Model file for the job. Use its own axes, mm. Face numbers are marked on the shaded views. A direction names the side the tool comes from. Give positions to 0.01 mm unless a question says otherwise; leave off trailing zeros. Loops run counter-clockwise (first coordinate to the right, second up) from the corner with the lowest first, then second, coordinate; pieces in that order, holes last. Notation, with made-up numbers: M -33.5,12.25 L -17.5,12.25 A20 ccw -17.5,33.25 Z; hole C -12,44.5 d10. An arc over 180 degrees is marked long. Answer in a Markdown table with one row per item.
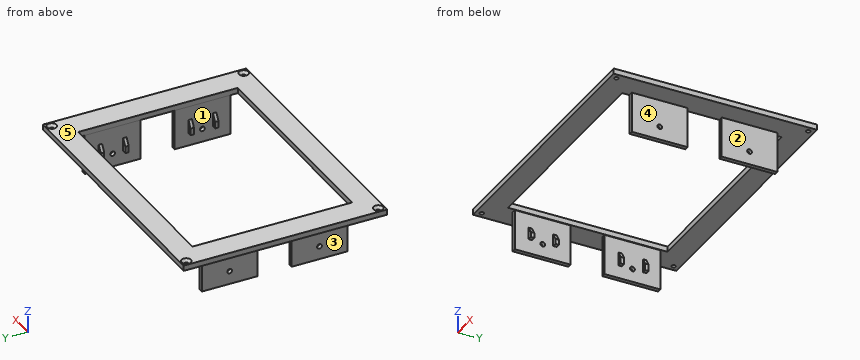
```python
from build123d import *
from OCP.BRepFilletAPI import BRepFilletAPI_MakeChamfer

# Parameters (mm, degrees)
ESQUISSE1_W             = 197
ESQUISSE1_H             = 149.5
BOSS_EXTRU_1_DEPTH      = 4
ESQUISSE3_R             = 1.5
ENL_V_MAT_EXTRU_2_DEPTH = 4
CHANFREIN1_SIZE         = 2
ESQUISSE4_W             = 160
ESQUISSE4_H             = 117.3
ENL_V_MAT_EXTRU_3_DEPTH = 10
ESQUISSE5_W             = 3
ESQUISSE5_H             = 41
BOSS_EXTRU_2_DEPTH      = 30
ESQUISSE6_W             = 10
ESQUISSE6_H             = 2.5
ESQUISSE6_W_2           = 8.882781921
BOSS_EXTRU_3_DEPTH      = 3
ESQUISSE7_W             = 10
ESQUISSE7_H             = 2.5
BOSS_EXTRU_4_DEPTH      = 3
CHANFREIN2_SIZE         = 3
CHANFREIN2_SIZE_2       = 5
ESQUISSE8_R             = 1.75
ENL_V_MAT_EXTRU_4_DEPTH = 210


with BuildPart() as part:
    # Esquisse1 → Boss.-Extru.1 (new body)
    with BuildSketch(Plane.XY):
        with Locations((98.5, 74.75)):
            Rectangle(ESQUISSE1_W, ESQUISSE1_H)
    extrude(amount=BOSS_EXTRU_1_DEPTH)

    # Esquisse3 → Enlèv. mat.-Extru.2 (cut)
    with BuildSketch(Plane.XY.offset(4)):
        with Locations((4.25, 145.25)):
            Circle(ESQUISSE3_R)
        with Locations((4.25, 4.25)):
            Circle(ESQUISSE3_R)
        with Locations((192.75, 4.25)):
            Circle(ESQUISSE3_R)
        with Locations((192.75, 145.25)):
            Circle(ESQUISSE3_R)
    extrude(amount=-ENL_V_MAT_EXTRU_2_DEPTH, mode=Mode.SUBTRACT)

    # Chanfrein1
    chanfrein1_edges = [part.edges().sort_by_distance(p)[0] for p in [
        (2.75, 145.25, 4),
        (2.75, 4.25, 4),
        (191.25, 4.25, 4),
        (191.25, 145.25, 4),
    ]]
    chamfer(chanfrein1_edges, length=CHANFREIN1_SIZE)

    # Esquisse4 → Enlèv. mat.-Extru.3 (cut)
    with BuildSketch(Plane.XY.offset(4)):
        with Locations((98.25, 74.75)):
            Rectangle(ESQUISSE4_W, ESQUISSE4_H)
    extrude(amount=-ENL_V_MAT_EXTRU_3_DEPTH, mode=Mode.SUBTRACT)

    # Esquisse5 → Boss.-Extru.2 (add)
    with BuildSketch(Plane(origin=(0, 0, 0), x_dir=(-1, 0, 0), z_dir=(0, 0, -1))):
        with Locations((-180.25, 107.9)):
            Rectangle(ESQUISSE5_W, ESQUISSE5_H)
        with Locations((-180.25, 41.9)):
            Rectangle(ESQUISSE5_W, ESQUISSE5_H)
        with Locations((-16.25, 107.9)):
            Rectangle(ESQUISSE5_W, ESQUISSE5_H)
        with Locations((-16.25, 41.9)):
            Rectangle(ESQUISSE5_W, ESQUISSE5_H)
    extrude(amount=BOSS_EXTRU_2_DEPTH)

    # Esquisse6 → Boss.-Extru.3 (add)
    with BuildSketch(Plane(origin=(17.75, 0, 0), x_dir=(0, 0, -1), z_dir=(1, 0, 0))):
        with Locations((15.5, 116.9)):
            Rectangle(ESQUISSE6_W, ESQUISSE6_H)
        with Locations((15.5, 98.9)):
            Rectangle(ESQUISSE6_W, ESQUISSE6_H)
        with Locations((14.941390961, 50.9)):
            Rectangle(ESQUISSE6_W_2, ESQUISSE6_H)
        with Locations((14.941390961, 32.9)):
            Rectangle(ESQUISSE6_W_2, ESQUISSE6_H)
    extrude(amount=BOSS_EXTRU_3_DEPTH)

    # Esquisse7 → Boss.-Extru.4 (add)
    with BuildSketch(Plane.ZY.offset(-178.75)):
        with Locations((-15.5, 32.9)):
            Rectangle(ESQUISSE7_W, ESQUISSE7_H)
        with Locations((-15.5, 50.9)):
            Rectangle(ESQUISSE7_W, ESQUISSE7_H)
        with Locations((-15.5, 98.9)):
            Rectangle(ESQUISSE7_W, ESQUISSE7_H)
        with Locations((-15.5, 116.9)):
            Rectangle(ESQUISSE7_W, ESQUISSE7_H)
    extrude(amount=BOSS_EXTRU_4_DEPTH)

    # Chanfrein2
    chanfrein2_edges_1 = [part.edges().sort_by_distance(p)[0] for p in [
        (20.75, 98.9, -10.5),
    ]]
    chanfrein2_side_1 = [part.faces().sort_by_distance(p)[0] for p in [
        (20.69, 98.9, -10.5),
    ]]
    chanfrein2_edges_2 = [part.edges().sort_by_distance(p)[0] for p in [
        (20.75, 116.9, -10.5),
    ]]
    chanfrein2_side_2 = [part.faces().sort_by_distance(p)[0] for p in [
        (20.69, 116.9, -10.5),
    ]]
    chanfrein2_edges_3 = [part.edges().sort_by_distance(p)[0] for p in [
        (20.75, 32.9, -10.5),
    ]]
    chanfrein2_side_3 = [part.faces().sort_by_distance(p)[0] for p in [
        (20.69, 32.9, -10.5),
    ]]
    chanfrein2_edges_4 = [part.edges().sort_by_distance(p)[0] for p in [
        (20.75, 50.9, -10.5),
    ]]
    chanfrein2_side_4 = [part.faces().sort_by_distance(p)[0] for p in [
        (20.69, 50.9, -10.5),
    ]]
    chanfrein2_edges_5 = [part.edges().sort_by_distance(p)[0] for p in [
        (175.75, 116.9, -10.5),
    ]]
    chanfrein2_side_5 = [part.faces().sort_by_distance(p)[0] for p in [
        (175.81, 116.9, -10.5),
    ]]
    chanfrein2_edges_6 = [part.edges().sort_by_distance(p)[0] for p in [
        (175.75, 98.9, -10.5),
    ]]
    chanfrein2_side_6 = [part.faces().sort_by_distance(p)[0] for p in [
        (175.81, 98.9, -10.5),
    ]]
    chanfrein2_edges_7 = [part.edges().sort_by_distance(p)[0] for p in [
        (175.75, 50.9, -10.5),
    ]]
    chanfrein2_side_7 = [part.faces().sort_by_distance(p)[0] for p in [
        (175.81, 50.9, -10.5),
    ]]
    chanfrein2_edges_8 = [part.edges().sort_by_distance(p)[0] for p in [
        (175.75, 32.9, -10.5),
    ]]
    chanfrein2_side_8 = [part.faces().sort_by_distance(p)[0] for p in [
        (175.81, 32.9, -10.5),
    ]]
    chanfrein2 = BRepFilletAPI_MakeChamfer(part.part.solid().wrapped)
    for e in chanfrein2_edges_1:
        chanfrein2.Add(CHANFREIN2_SIZE - 0.0001, CHANFREIN2_SIZE_2 - 0.0001, e.wrapped, chanfrein2_side_1[0].wrapped)
    for e in chanfrein2_edges_2:
        chanfrein2.Add(CHANFREIN2_SIZE - 0.0001, CHANFREIN2_SIZE_2 - 0.0001, e.wrapped, chanfrein2_side_2[0].wrapped)
    for e in chanfrein2_edges_3:
        chanfrein2.Add(CHANFREIN2_SIZE - 0.0001, CHANFREIN2_SIZE_2 - 0.0001, e.wrapped, chanfrein2_side_3[0].wrapped)
    for e in chanfrein2_edges_4:
        chanfrein2.Add(CHANFREIN2_SIZE - 0.0001, CHANFREIN2_SIZE_2 - 0.0001, e.wrapped, chanfrein2_side_4[0].wrapped)
    for e in chanfrein2_edges_5:
        chanfrein2.Add(CHANFREIN2_SIZE - 0.0001, CHANFREIN2_SIZE_2 - 0.0001, e.wrapped, chanfrein2_side_5[0].wrapped)
    for e in chanfrein2_edges_6:
        chanfrein2.Add(CHANFREIN2_SIZE - 0.0001, CHANFREIN2_SIZE_2 - 0.0001, e.wrapped, chanfrein2_side_6[0].wrapped)
    for e in chanfrein2_edges_7:
        chanfrein2.Add(CHANFREIN2_SIZE - 0.0001, CHANFREIN2_SIZE_2 - 0.0001, e.wrapped, chanfrein2_side_7[0].wrapped)
    for e in chanfrein2_edges_8:
        chanfrein2.Add(CHANFREIN2_SIZE - 0.0001, CHANFREIN2_SIZE_2 - 0.0001, e.wrapped, chanfrein2_side_8[0].wrapped)
    add(Compound.cast(chanfrein2.Shape()), mode=Mode.REPLACE)  # a hair under: the kernel refuses the full size

    # Esquisse8 → Enlèv. mat.-Extru.4 (cut)
    with BuildSketch(Plane.ZY.offset(-14.75)):
        with Locations(Location((-20.25, 107.9, 0), (0, 0, 270))):
            Circle(ESQUISSE8_R)
        with Locations(Location((-20.25, 41.9, 0), (0, 0, 270))):
            Circle(ESQUISSE8_R)
    extrude(amount=-ENL_V_MAT_EXTRU_4_DEPTH, mode=Mode.SUBTRACT)


solid = part.part
```
(1) Wall check: L1, parallel to X at y = 145.25, z = 1.15; L2, parallel to Z at x = 180.6, y = 107.9; L3, parallel to X at y = 54, z = -20. Give the ranges that are in metal, low to high.
Established:
| item | result |
|---|---|
| L1 | x = 0 to 2.75, 5.75 to 191.25, 194.25 to 197 |
| L2 | z = -30 to -22, -18.5 to 4 |
| L3 | x = 14.75 to 17.75, 178.75 to 181.75 |
(2) Which spindle directions (+Z, -Z, +X, -X, +Y, -Y) get a long thin tool onto all of the face, cutting with end or side? Do the marked faces 3, 4 and 5. Say none if no direction does.
Established:
| item | result |
|---|---|
| face 3 | -Z, -X, +Y, -Y |
| face 4 | -Z, +X, +Y, -Y |
| face 5 | +Z, +X, -X, +Y, -Y |
(3) Saw through at A-A, the plane x = 27. Give the cut face in (y, z).
Established:
| item | result |
|---|---|
| outline | M 0,0 L 16.1,0 L 16.1,4 L 0,4 Z; M 133.4,0 L 149.5,0 L 149.5,4 L 133.4,4 Z |
(4) Saw through at B-B, the plane z = -26. Give the cut face in (x, y).
Established:
| item | result |
|---|---|
| outline | M 14.75,21.4 L 17.75,21.4 L 17.75,62.4 L 14.75,62.4 Z; M 14.75,87.4 L 17.75,87.4 L 17.75,128.4 L 14.75,128.4 Z; M 178.75,21.4 L 181.75,21.4 L 181.75,62.4 L 178.75,62.4 Z; M 178.75,87.4 L 181.75,87.4 L 181.75,128.4 L 178.75,128.4 Z |
(5) Mould opens along Y. For the marked faces 1 and 2 say: pulls with the +Y half, pulls with the -Y half, needs draft (parallel to the pull), parting line crosses it, or undercut.
Established:
| item | result |
|---|---|
| face 1 | undercut |
| face 2 | needs draft |
(6) Flat gauge pins, fed straight in: P1, Ø12, axis at x = 141, y = 19, coming from the -Z side; P2, Ø4.5, axis at y = 41.9, z = -20.25, coming from the +X side; P3, Ø4, axis at x = 4.25, y = 4.25, coming from the +Z side. Where does each tip first touch, or does it go through?
Established:
| item | result |
|---|---|
| P1 | stops at z = 0 |
| P2 | stops at x = 181.75 |
| P3 | stops at z = 2.5 |
